Autodesk Inventor part; units mm, degrees
ref_plane "YZ Plane" through (0, 0, 0) normal (1, 0, 0) x (0, 1, 0)
ref_plane "XZ Plane" through (0, 0, 0) normal (0, 1, 0) x (-1, 0, 0)
ref_plane "XY Plane" through (0, 0, 0) normal (0, 0, 1) x (1, 0, 0)
sketch "Sketch1" plane through (0, 0, 0) normal (0, 0, 1) x (1, 0, 0)
  circle A0 centre (0, 0) radius 22.5
  dimension "d0" = 45
extrude "Extrusion1" add sketch "Sketch1" along normal blind 100
sketch "Sketch2" plane through (0, 0, 0) normal (0, 0, -1) x (-1, 0, 0)
  circle A0 centre (0, 0) radius 17.5
  point P0 (-6.0869, 16.4073)
  point P1 (4.042, 17.0268)
  point P2 (5, 16.7705)
  point P3 (-5, 16.7705)
  dimension "d3" = 35
sketch "Sketch5" plane through (0, 0, 100) normal (0, 0, 1) x (1, 0, 0)
  line L0 (-75, -10) -> (75, -10)
  line L1 (75, -10) -> (75, 10)
  line L2 (75, 10) -> (-75, 10)
  line L3 (-75, 10) -> (-75, -10)
  line L4 (-75, -10) -> (75, 10) construction
  line L5 (75, -10) -> (-75, 10) construction
  point P0 (0, 0)
  dimension "d32" = 150
  dimension "d33" = 20
extrude "Extrusion5" add sketch "Sketch5" along normal blind 150
sketch "Sketch8" plane through (0, 0, 250) normal (0, 0, 1) x (1, 0, 0)
  circle A0 centre (0, 0) radius 22.5
  dimension "d136" = 45
extrude "Extrusion8" add sketch "Sketch8" along normal blind 100
sketch "Sketch11" plane through (-20.1556, 10, 100) normal (0, 1, 0) x (1, 0, 0)
  line L0 (-44.8444, -140) -> (85.1556, -140)
  line L1 (85.1556, -140) -> (85.1556, -10)
  line L2 (85.1556, -10) -> (-44.8444, -10)
  line L3 (-44.8444, -10) -> (-44.8444, -140)
  line L4 (-44.8444, -140) -> (85.1556, -10) construction
  line L5 (85.1556, -140) -> (-44.8444, -10) construction
  line L6 (-54.8444, 0) -> (-54.8444, -150)
  line L7 (0, -150) -> (40.3113, -150)
  line L8 (-54.8444, -127.249) -> (-44.8444, -127.249)
  line L9 (-54.8444, -150) -> (0, -150)
  line L10 (-32.0934, -150) -> (-32.0934, -140)
  line L11 (-54.8444, 0) -> (-54.8444, -150)
  line L12 (-54.8444, -22.751) -> (-44.8444, -22.751)
  line L13 (-32.0934, 0) -> (-32.0934, -10)
  line L14 (0, 0) -> (40.3113, 0)
  line L15 (72.4046, 0) -> (72.4046, -10)
  line L16 (95.1556, -22.751) -> (85.1556, -22.751)
  line L17 (40.3113, -150) -> (95.1556, -150)
  line L18 (72.4046, -150) -> (72.4046, -140)
  line L19 (95.1556, 0) -> (95.1556, -150)
  line L20 (95.1556, -127.249) -> (85.1556, -127.249)
  line L21 (-44.8444, -75) -> (-44.8444, -40)
  line L22 (-44.8444, -75) -> (-44.8444, -110)
  line L23 (-44.8444, -40) -> (-31.8444, -40)
  line L24 (20.1556, -10) -> (-14.8444, -10)
  line L25 (20.1556, -10) -> (55.1556, -10)
  line L26 (-14.8444, -10) -> (-14.8444, -23)
  arc A0 (-14.8444, -23) -> (-31.8444, -40) centre (21.321, -76.1654) ccw
  line L27 (20.1556, -140) -> (-14.8444, -140)
  line L28 (20.1556, -140) -> (55.1556, -140)
  line L29 (85.1556, -75) -> (85.1556, -110)
  line L30 (85.1556, -75) -> (85.1556, -40)
  line L31 (20.1556, -10) -> (55.1556, -10)
  line L32 (-44.8444, -110) -> (-31.8444, -110)
  line L33 (-14.8444, -140) -> (-14.8444, -127)
  line L34 (55.1556, -140) -> (55.1556, -127)
  line L35 (85.1556, -110) -> (72.1556, -110)
  line L36 (85.1556, -40) -> (72.1556, -40)
  line L37 (55.1556, -10) -> (55.1556, -23)
  arc A1 (55.1556, -127) -> (72.1556, -110) centre (18.9903, -73.8346) ccw
  arc A2 (-31.8444, -110) -> (-14.8444, -127) centre (21.321, -73.8346) ccw
  arc A3 (72.1556, -40) -> (55.1556, -23) centre (18.9903, -76.1654) ccw
  point P0 (20.1556, 100)
  point P1 (20.1556, -75)
  dimension "d72" = 130
  dimension "d73" = 130
  dimension "d74" = 75
  dimension "d75" = 75
  dimension "d84" = 35
  dimension "d85" = 35
  dimension "d86" = 13
  dimension "d87" = 35
  dimension "d88" = 35
  dimension "d89" = 13
  dimension "d90" = 64.3
  dimension "d96" = 35
  dimension "d97" = 35
  dimension "d98" = 35
  dimension "d99" = 35
  dimension "d100" = 13
  dimension "d101" = 13
  dimension "d102" = 13
  dimension "d103" = 13
  dimension "d104" = 13
  dimension "d105" = 13
  dimension "d106" = 64.3
  dimension "d107" = 64.3
  dimension "d108" = 64.3
extrude "Extrusion10" cut sketch "Sketch11" against normal blind 20 contours L33 A2 L32 L3 L23 A0 L26 L2 L37 A3 L36 L1 L35 A1 L34 L0
sketch "Sketch12" plane through (-20.1556, 10, 100) normal (0, 1, 0) x (1, 0, 0)
  circle A0 centre (-31.1094, -27.235) radius 4.5
  line L0 (-44.8444, -40) -> (-31.8444, -40)
  line L1 (-44.8444, -110) -> (-44.8444, -40)
  circle A1 centre (-31.1094, -122.765) radius 4.5
  circle A2 centre (71.4206, -122.765) radius 4.5
  circle A3 centre (71.4206, -27.235) radius 4.5
  line L2 (-31.8444, -110) -> (-44.8444, -110)
  line L3 (85.1556, -110) -> (72.1556, -110)
  line L4 (85.1556, -40) -> (85.1556, -110)
  line L5 (72.1556, -40) -> (85.1556, -40)
  point P0 (20.1556, 100)
  point P1 (-28.3394, -127.249)
  dimension "d91" = 9
  dimension "d92" = 12.765
  dimension "d93" = 13.735
  dimension "d109" = 9
  dimension "d110" = 9
  dimension "d111" = 9
  dimension "d112" = 12.765
  dimension "d113" = 13.735
  dimension "d114" = 12.765
  dimension "d115" = 13.735
  dimension "d116" = 13.735
  dimension "d117" = 12.765
extrude "Extrusion11" cut sketch "Sketch12" along normal mid plane 50
sketch "Sketch13" plane through (-20.1556, 10, 100) normal (0, 1, 0) x (1, 0, 0)
  line L0 (-44.8444, -110) -> (-44.8444, -40)
  line L1 (55.1556, -140) -> (-14.8444, -140)
  arc A0 (-44.8444, -110) -> (-14.8444, -140) centre (-20.4902, -115.6459) ccw
  line L2 (-14.8444, -10) -> (-14.8444, -23)
  arc A1 (-14.8444, -10) -> (-44.8444, -40) centre (-20.4902, -34.3541) ccw
  line L3 (85.1556, -110) -> (85.1556, -40)
  arc A2 (55.1556, -140) -> (85.1556, -110) centre (60.8015, -115.6459) ccw
  line L4 (85.1556, -40) -> (72.1556, -40)
  line L5 (55.1556, -23) -> (55.1556, -10)
  arc A3 (85.1556, -40) -> (55.1556, -10) centre (60.8015, -34.3541) ccw
  line L6 (-14.8444, -127) -> (-14.8444, -140)
  line L7 (-14.8444, -140) -> (-14.8444, -127)
  arc A4 (-31.8444, -110) -> (-14.8444, -127) centre (21.321, -73.8346) ccw
  line L8 (-44.8444, -110) -> (-31.8444, -110)
  arc A5 (-31.8444, -110) -> (-14.8444, -127) centre (21.321, -73.8346) ccw
  line L9 (-31.8444, -40) -> (-44.8444, -40)
  line L10 (-44.8444, -40) -> (-31.8444, -40)
  line L11 (-14.8444, -10) -> (-14.8444, -23)
  line L12 (55.1556, -10) -> (55.1556, -23)
  line L13 (72.1556, -40) -> (85.1556, -40)
  line L14 (85.1556, -110) -> (72.1556, -110)
  line L15 (72.1556, -110) -> (85.1556, -110)
  arc A6 (-14.8444, -23) -> (-31.8444, -40) centre (21.321, -76.1654) ccw
  arc A7 (-14.8444, -23) -> (-31.8444, -40) centre (21.321, -76.1654) ccw
  arc A8 (72.1556, -40) -> (55.1556, -23) centre (18.9903, -76.1654) ccw
  line L16 (55.1556, -140) -> (55.1556, -127)
  line L17 (55.1556, -140) -> (55.1556, -127)
  arc A9 (55.1556, -127) -> (72.1556, -110) centre (18.9903, -73.8346) ccw
  arc A10 (55.1556, -127) -> (72.1556, -110) centre (18.9903, -73.8346) ccw
  point P0 (20.1556, 100)
  dimension "d118" = 25
  dimension "d119" = 25
  dimension "d120" = 25
  dimension "d121" = 25
  dimension "d122" = 64.3
  dimension "d125" = 64.3
  dimension "d126" = 64.3
  dimension "d127" = 64.3
extrude "Extrusion12" add sketch "Sketch13" along normal blind 30
sketch "Sketch14" plane through (-20.1556, -10, 100) normal (0, -1, 0) x (1, 0, 0)
  circle A0 centre (-31.1094, 27.235) radius 4.5
  circle A1 centre (-31.1094, 27.235) radius 4.5
  circle A2 centre (-31.1094, 122.765) radius 4.5
  circle A3 centre (-31.1094, 122.765) radius 4.5
  circle A4 centre (71.4206, 122.765) radius 4.5
  circle A5 centre (71.4206, 122.765) radius 4.5
  circle A6 centre (71.4206, 27.235) radius 4.5
  circle A7 centre (71.4206, 27.235) radius 4.5
  point P0 (20.1556, -100)
  dimension "d130" = 9
  dimension "d131" = 9
  dimension "d132" = 9
  dimension "d133" = 9
extrude "Extrusion13" cut sketch "Sketch14" against normal blind 100
extrude "Extrusion14" cut sketch "Sketch2" against normal blind 76
fillet "Fillet7" radius 7.62 8 edges at (65, 0, 210) (65, 0, 140) (35, 0, 110) (35, 0, 240) (-35, 0, 240) (-65, 0, 210) (-65, 0, 140) (-35, 0, 110)
equation "\"d84\" = d98"
equation "\"d85\" = d98"
equation "\"d86\" = d104"
equation "\"d87\" = d98"
equation "\"d88\" = d98"
equation "\"d89\" = d104"
equation "\"d96\" = d98"
equation "\"d97\" = d98"
equation "\"d99\" = d98"
equation "\"d100\" = d104"
equation "\"d101\" = d104"
equation "\"d102\" = d105"
equation "\"d103\" = d104"
equation "\"d112\" = d92"
equation "\"d113\" = d93"
equation "\"d114\" = d112"
equation "\"d115\" = d113"
equation "\"d116\" = d115"
equation "\"d117\" = d114"
properties part number "FrontPlateV2"
Source: CAD feature listing. Evaluate the final solid. Frame: model axes, mm. A direction names the side the tool comes from. Coordinates: 2 decimals unless noted, no trailing zeros. Loops run counter-clockwise (first coordinate to the right, second up) from the corner with the lowest first, then second, coordinate; pieces in that order, holes last. Notation, with made-up numbers: M 74,26.25 L 126,26.25 A24 ccw 126,57.25 Z; hole C 25,79 d4. An arc over 180 degrees is marked long. Answer in a Markdown table with one row per item.
Q1. First-contact query: pin 1 (6 mm diameter, centred on x = -23.5, z = 99.5, fed in from -Y); pin 2 (22 mm diameter, centred on x = -58, y = -2, fed in from -Z); pin 3 (1.5 mm diameter, centred on x = 17, z = 296, fed in from +Y). Flat tips, straight axial feed; report the tip coordinate or a pass-through.
Answers below:
| item | result |
|---|---|
| pin 1 | stops at y = -10 |
| pin 2 | stops at z = 100 |
| pin 3 | stops at y = 15.56 |
Q2. Section A-A on y = 32.5. Return the cut outline in (x, z) (3 decimals).
Answers below:
| item | result |
|---|---|
| outline | M -63.865,143.62 A25 ccw -31.38,111.135 A7.62 cw -35,117.62 L -35,123 A64.3 cw -52,140 L -57.38,140 A7.62 cw Z; M -63.865,206.38 A7.62 cw -57.38,210 L -52,210 A64.3 cw -35,227 L -35,232.38 A7.62 cw -31.38,238.865 A25 ccw Z; M 31.38,111.135 A25 ccw 63.865,143.62 A7.62 cw 57.38,140 L 52,140 A64.301 cw 35,123 L 35,117.62 A7.62 cw Z; M 31.38,238.865 A7.62 cw 35,232.38 L 35,227 A64.299 cw 52,210 L 57.38,210 A7.62 cw 63.865,206.38 A25 ccw Z; hole C -51.265,127.235 d9; hole C -51.265,222.765 d9; hole C 51.265,127.235 d9; hole C 51.265,222.765 d9 |
Q3. Ray query, probe 1 along Z at (x, y) = (-25, 5.5); probe 2 along Z at (x, y) = (9, 17); probe 3 along X at (y, z) = (3.5, 148). Return the intervals inside material, ascending. Write a range as from..to.
Answers below:
| item | result |
|---|---|
| probe 1 | z = 100..110, 240..250 |
| probe 2 | z = 0..100, 250..350 |
| probe 3 | x = -75..-65, 65..75 |
Q4. Set-up query: faces 1 (the flat face through (0, 15, 250)), 2 (the flat face through (1, 10, 241)), 3 (the cylindrical face through (-44.421, 15.35, 219.182)), 4 (the flat face through (12, -13, 0)). Return all of +Z, -Z, +X, -X, +Y, -Y with unobstructed straight access to the full face (end or side cutting, diameter ignored); none if empty.
Answers below:
| item | result |
|---|---|
| face 1 | +X, -X, +Y |
| face 2 | +Y |
| face 3 | +Y, -Y |
| face 4 | -Z, +X, -X, +Y, -Y |
Q5. Draft query along X for faces 5 (the cylindrical face through (-33.67, 15.35, 236.68)), 6 (the flat face through (-49, 40, 122)), 7 (the cylindrical face through (44.421, 15.35, 130.818)). Return one class per face: pulls with the +X half, pulls with the -X half, needs draft (parallel to the pull), parting line crosses it, or undercut.
Answers below:
| item | result |
|---|---|
| face 5 | undercut |
| face 6 | needs draft |
| face 7 | undercut |
Q6. Section B-B on x = 0. Return the cut outline in (y, z).
Answers below:
| item | result |
|---|---|
| outline | M -22.5,0 L -17.5,0 L -17.5,76 L 17.5,76 L 17.5,0 L 22.5,0 L 22.5,100 L 10,100 L 10,110 L -10,110 L -10,100 L -22.5,100 Z; M -22.5,250 L -10,250 L -10,240 L 10,240 L 10,250 L 22.5,250 L 22.5,350 L -22.5,350 Z |
Q7. Section D-D on y = -14. Return the cut outline in (x, z), plus the area to 3 significant figures.
Answers below:
| item | result |
|---|---|
| outline | M -17.61,0 L -10.5,0 L -10.5,76 L 10.5,76 L 10.5,0 L 17.61,0 L 17.61,100 L -17.61,100 Z; M -17.61,250 L 17.61,250 L 17.61,350 L -17.61,350 Z |
| area | 5,450 mm^2 |
Q8. Section C-C on z = 184.5. Return the cut outline in (x, y).
Answers below:
| item | result |
|---|---|
| outline | M -75,-10 L -65,-10 L -65,10 L -75,10 Z; M 65,-10 L 75,-10 L 75,10 L 65,10 Z |
